Part model, mm, in its own coordinate system. Round coordinates to 2 decimals unless told otherwise and drop trailing zeros. Write each loop counter-clockwise with the first axis right and the second up, starting at its lowest first coordinate (ties: lowest second). Pieces come first, ordered by that corner, then holes.
```python
from build123d import *

# Parameters (mm, degrees)
F1_DEPTH = 1000
F2_R     = 3.5
F3_R     = 7


with BuildPart() as f1:
    # F0 (on Top) → F1 (new body)
    with BuildSketch(Plane.XY):
        Polygon((-20, 17.5), (-20, -17.5), (20, -17.5), (20, 17.5), (14.400024, 17.5), (11.999983, -12.5), (-11.999983, -12.5), (-14.400024, 17.5), align=None)
    extrude(amount=-F1_DEPTH)

    # F2
    f2_edges = [f1.edges().sort_by_distance(p)[0] for p in [
        (-14.400024, 17.5, -500),
        (14.400024, 17.5, -500),
    ]]
    fillet(f2_edges, radius=F2_R)

    # F3
    f3_edges = [f1.edges().sort_by_distance(p)[0] for p in [
        (-11.999983, -12.5, -500),
        (11.999983, -12.5, -500),
    ]]
    fillet(f3_edges, radius=F3_R)


solid = f1.part
```
Q1. Wall check: L1, parallel to X at y = 14.5, z = -281; L2, parallel to X at y = -5.5, z = -138; L3, parallel to Y at x = 6.5, z = -123.5. Give the ranges that are in metal, low to high.
Values follow:
L1: x = -20 to -14.17, 14.17 to 20
L2: x = -20 to -12.56, 12.56 to 20
L3: y = -17.5 to -12.43
Q2. Drop flat-ended pins along their axis: pin 1 (1.5 mm diameter, centred on x = 2.5, y = -12.5, fed in from +Z); pin 2 (5.5 mm diameter, centred on x = -1.5, z = -268.5, fed in from +Y). Give the stop position or say it passes through.
Values follow:
pin 1: stops at z = 0
pin 2: stops at y = -12.5
Q3. Cut at A-A on z = -791. Write the cut outline in (x, y), plus the area to 3 significant figures.
Values follow:
outline: (-20, -17.5) - (20, -17.5) - (20, 17.5) - (17.63, 17.5) arc R3.5 ccw to (14.14, 14.28) - (12.52, -6.06) arc R7 cw to (5.54, -12.5) - (-5.54, -12.5) arc R7 cw to (-12.52, -6.06) - (-14.14, 14.28) arc R3.5 ccw to (-17.63, 17.5) - (-20, 17.5) - close
area: 621 mm2
Q4. Mould opens along X. For faces 1 (the flat face through (13.34, 4.25, -493)), 2 (the flat face through (-20, 0, -493)), 3 (the flat face through (-13.317, 3.968, -493)), 4 (the flat face through (0, -15, -1000)) say: +X half, -X half, draft (parallel to the pull), parting line (faces both ways), or undercut.
Values follow:
face 1: undercut
face 2: -X half
face 3: undercut
face 4: draft
